```python
from build123d import *

# Parameters (mm, degrees)
SCHIZZO1_W                   = 449
SCHIZZO1_H                   = 94
SCHIZZO1_R                   = 7.8
SCHIZZO1_R_2                 = 2
ESTRUSIONE_ESTRUSIONE1_DEPTH = 4


with BuildPart() as part:
    # Schizzo1 → Estrusione-Estrusione1 (new body)
    with BuildSketch(Plane.XY):
        with Locations((-224.5, 47)):
            Rectangle(SCHIZZO1_W, SCHIZZO1_H)
        with Locations(Location((-384, 27, 0), (0, 0, 180))):
            Circle(SCHIZZO1_R, mode=Mode.SUBTRACT)
        with Locations((-9, 47)):
            Circle(SCHIZZO1_R_2, mode=Mode.SUBTRACT)
        with Locations((-224.5, 85)):
            Circle(SCHIZZO1_R_2, mode=Mode.SUBTRACT)
        with Locations(Location((-440, 47, 0), (0, 0, 180))):
            Circle(SCHIZZO1_R_2, mode=Mode.SUBTRACT)
        with Locations(Location((-224.5, 9, 0), (0, 0, 180))):
            Circle(SCHIZZO1_R_2, mode=Mode.SUBTRACT)
        with Locations((-324, 27)):
            Circle(SCHIZZO1_R, mode=Mode.SUBTRACT)
        with Locations(Location((-324, 67, 0), (0, 0, 180))):
            Circle(SCHIZZO1_R, mode=Mode.SUBTRACT)
        with Locations((-336.75, 85)):
            Circle(SCHIZZO1_R_2, mode=Mode.SUBTRACT)
        with Locations((-384, 67)):
            Circle(SCHIZZO1_R, mode=Mode.SUBTRACT)
        with Locations(Location((-336.75, 9, 0), (0, 0, 180))):
            Circle(SCHIZZO1_R_2, mode=Mode.SUBTRACT)
        with Locations((-112.25, 9)):
            Circle(SCHIZZO1_R_2, mode=Mode.SUBTRACT)
        with Locations(Location((-112.25, 85, 0), (0, 0, 180))):
            Circle(SCHIZZO1_R_2, mode=Mode.SUBTRACT)
    extrude(amount=ESTRUSIONE_ESTRUSIONE1_DEPTH)


solid = part.part
```
CAD build for the part. Positions are in the model's coordinates, mm. Give positions to 0.01 mm unless a question says otherwise; leave off trailing zeros. Write each loop counter-clockwise with the first axis right and the second up, starting at its lowest first coordinate (ties: lowest second). Pieces come first, ordered by that corner, then holes. Notation, with made-up numbers: M 69.25,-22.5 L 115.25,-22.5 A27 cw 115.25,-3.5 Z; hole C 53.5,24.5 d9. An arc over 180 degrees is marked long. Return JSON: item names as keys, results as strings. Group by question number.
(1) Band-saw the part on B-B (z = 1.8). State how many separate pieces and enclosed holes the cut face has, and give its area (3 significant figures).
(2) Drill centre lines: L1, parallel to Y at x = -324, z = 1.05; L2, parallel to Y at x = -112.25, z = 1.95; L3, parallel to X at y = 46.5, z = 0.25. Where is each one in solid material? Low to high. Write a range as [from, to].
(3) Mould opens along Y. For faces 1 (the face through (-390.19, 62.254, 1.972)), 2 (the face through (-228, 48, 4)) say: pulls with the +Y half, pulls with the -Y half, needs draft (parallel to the pull), parting line crosses it, or undercut.
(4) Band-saw the part on A-A (x = -324). Give the cut face in (y, z), and give its area (3 significant figures).
(5) Band-saw the part on C-C (y = 67). Give the cut face in (x, z), and give its area (3 significant figures).
Entries:
{
 "1": {"separate pieces": "1", "enclosed holes": "12", "area": "41,300 mm^2"},
 "2": {"L1": "y = [0, 19.2], [34.8, 59.2], [74.8, 94]", "L2": "y = [0, 7], [11, 83], [87, 94]", "L3": "x = [-449, -441.94], [-438.06, -10.94], [-7.06, 0]"},
 "3": {"face 1": "undercut", "face 2": "needs draft"},
 "4": {"outline": "M 0,0 L 19.2,0 L 19.2,4 L 0,4 Z; M 34.8,0 L 59.2,0 L 59.2,4 L 34.8,4 Z; M 74.8,0 L 94,0 L 94,4 L 74.8,4 Z", "area": "251 mm^2"},
 "5": {"outline": "M -449,0 L -391.8,0 L -391.8,4 L -449,4 Z; M -376.2,0 L -331.8,0 L -331.8,4 L -376.2,4 Z; M -316.2,0 L 0,0 L 0,4 L -316.2,4 Z", "area": "1,670 mm^2"}
}
